Design review of the part shown in the three views and the two pictorial views. Dimensions are in mm from the part's minimum x, y and z. A direction names the side the tool comes from. Round coordinates to 2 decimals unless told otherwise and drop trailing zeros. Order: outer loops, then holes, each group sorted by start corner. A loop starts at its lowest first (then second) coordinate and runs counter-clockwise, first axis right, second up. Notation, with made-up numbers: (-18.75, -19.75) - (6.25, -19.75) arc R18 ccw to (6.25, 7.25) - close; hole circle Ø2 at (45.5, 77). An arc over 180 degrees is marked (long way). Use CSV: the item, a comma, the result in double quotes.
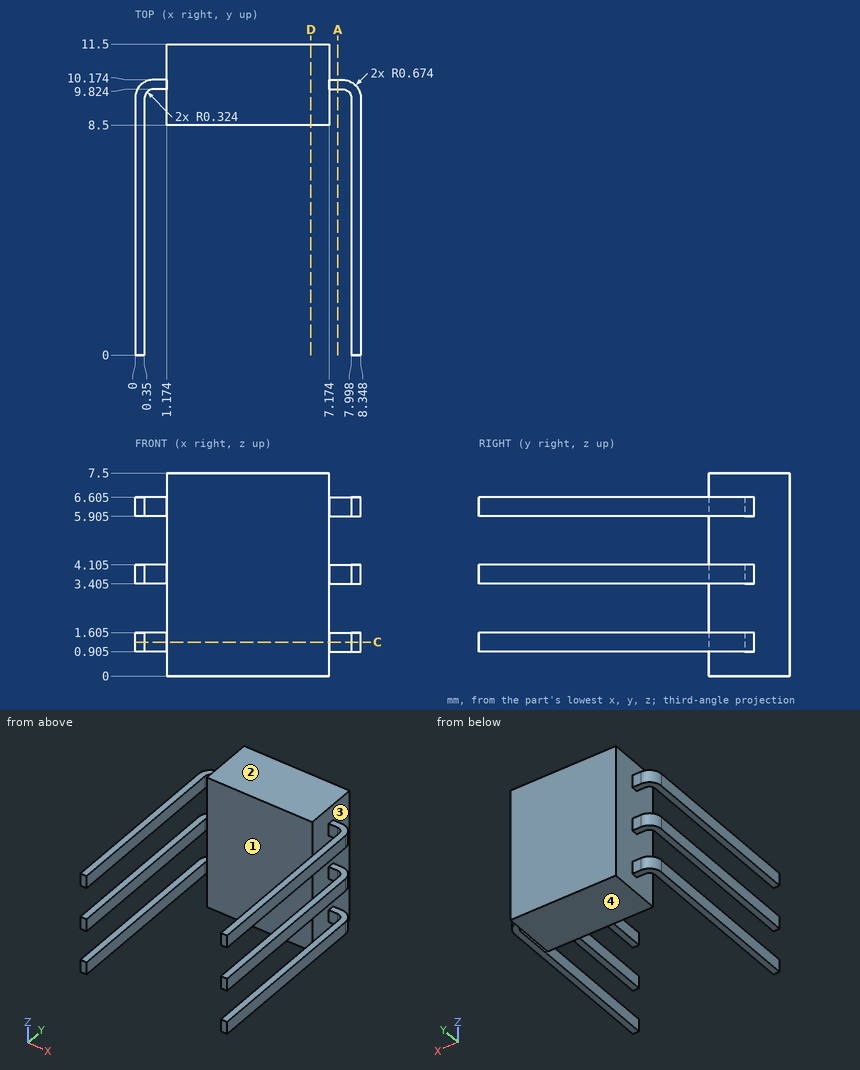
1) The part is to be moulded in two halves that separate along X. For the marked faces 3 and 4, say which applies: +X half, -X half, draft (parallel to the pull), parting line (faces both ways), or undercut.
Data:
face 3,"undercut"
face 4,"draft"
2) Insertion check: pin 1 Ø2 at (x, z) = (3.5, 6) entering from -Y; pin 2 Ø0.9 at (x, y) = (0.5, 5) entering from -Z (1 decimal); pin 3 Ø0.9 at (y, z) = (10.5, 2) entering from -X. Each pin has a flat end and moves straight along its axis. Give the tip position at first contact, or say it passes through.
Data:
pin 1,"stops at y = 8.5"
pin 2,"stops at z = 0.9"
pin 3,"stops at x = 1.17"
3) We need section D-D (x = 6.5). Give the boundary of the cut face in (y, z).
Data:
outline,"(8.5, 0) - (11.5, 0) - (11.5, 7.5) - (8.5, 7.5) - close"
4) For the marked faces 1 and 2, list the 3-axis set-ups (+Z, -Z, +X, -X, +Y, -Y) from which the entire face can be reached by the end or side of a thin tool; tool diameter is ignored.
Data:
face 1,"+Z, -Z, -Y"
face 2,"+Z, +X, -X, +Y, -Y"
5) We need section A-A (x = 7.5). Give the number of separate pieces and of enclosed holes in the cut face.
Data:
separate pieces,"3"
enclosed holes,"0"
6) We need section C-C (z = 1.25). Give the boundary of the cut face in (x, y).
Data:
outline,"(0, 0) - (0.35, 0) - (0.35, 9.5) arc R0.32 cw to (0.67, 9.82) - (1.17, 9.82) - (1.17, 8.5) - (7.17, 8.5) - (7.17, 9.82) - (7.67, 9.82) arc R0.32 cw to (8, 9.5) - (8, 0) - (8.35, 0) - (8.35, 9.5) arc R0.67 ccw to (7.67, 10.17) - (7.17, 10.17) - (7.17, 11.5) - (1.17, 11.5) - (1.17, 10.17) - (0.67, 10.17) arc R0.67 ccw to (0, 9.5) - close"
7) To check wall thickness, follow L1, parallel to X at y = 9.5, z = 3.5; L2, parallel to X at y = 1.5, z = 3.5; L3, parallel to Y at x = 3.5, z = 5.75. State the ranges of each line that lie inside material, in increasing order. Write a range as from..to.
Data:
L1,"x = 0..0.35, 1.17..7.17, 8..8.35"
L2,"x = 0..0.35, 8..8.35"
L3,"y = 8.5..11.5"
